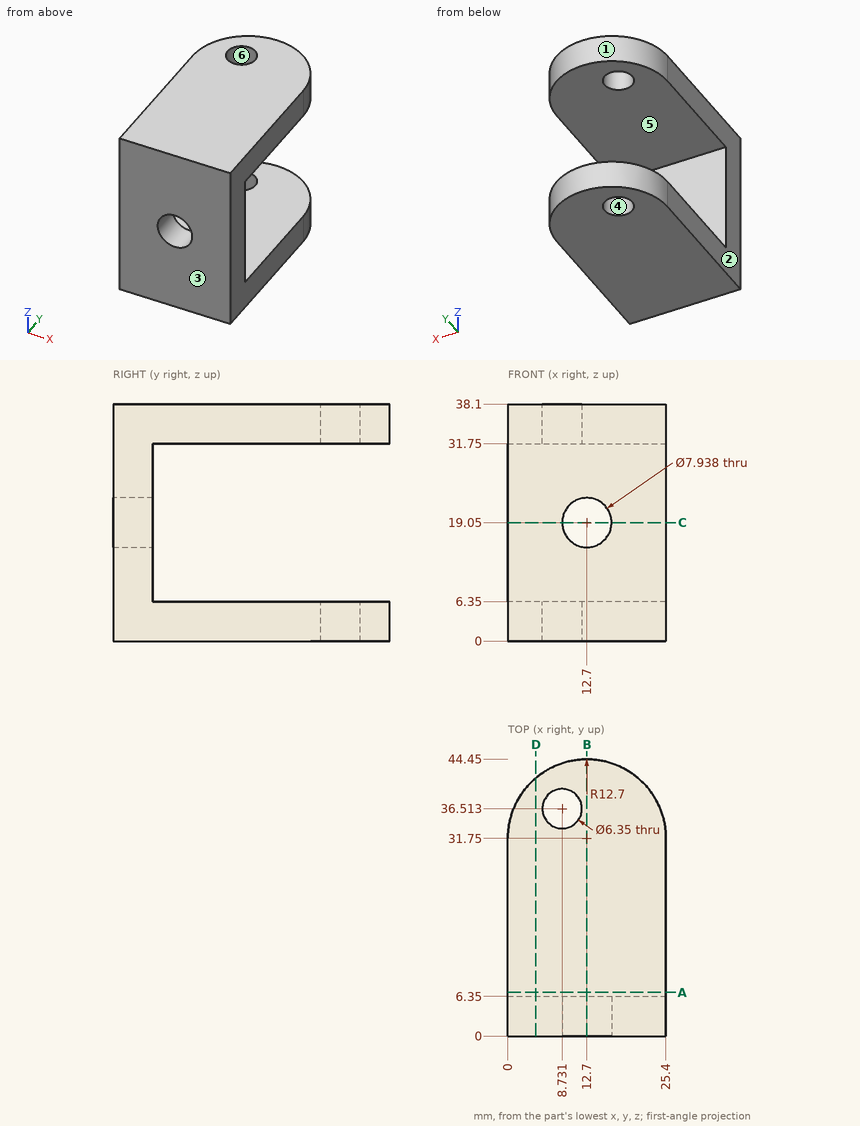
Geometry: see drawing. Coordinates: mm, zero at the bounding-box minimum. A direction names the side the tool comes from. Round coordinates to 2 decimals unless told otherwise and drop trailing zeros. Write each loop counter-clockwise with the first axis right and the second up, starting at its lowest first coordinate (ties: lowest second). Pieces come first, ordered by that corner, then holes.
1) Reachability of the marked faces 5 and 6 from +Z, -Z, +X, -X, +Y, -Y: full face, straight path, thin tool, end or side. Return the list, or none.
2) Draft query along X for the marked faces 1, 2, 3 and 4. Return one class per face: pulls with the +X half, pulls with the -X half, needs draft (parallel to the pull), parting line crosses it, or undercut.
3) Cut plane B-B (x = 12.7). Return the cut outline in (y, z).
4) Ray query, L1, parallel to Z at x = 12.25, y = 11; L2, parallel to X at y = 4.5, z = 19.05; L3, parallel to Y at x = 23, z = 24. Return the intervals inside material, ascending.
5) Cut plane C-C (z = 19.05). Return the cut outline in (x, y).
6) Contact query for a flat-ended pin moving along its axis: P1, Ø5, axis at x = 17, z = 29.5, coming from the +Y side. Output: stop coordinate, or through.
7) Cut plane D-D (x = 4.5). Return the cut outline in (y, z).
8) Cut plane A-A (y = 7). Return the cut outline in (x, z).
Geometry says:
1. face 5: +X, -X, +Y
1. face 6: +Z, -Z
2. face 1: parting line crosses it
2. face 2: pulls with the -X half
2. face 3: needs draft
2. face 4: undercut
3. outline: (0, 0) - (44.45, 0) - (44.45, 6.35) - (6.35, 6.35) - (6.35, 15.08) - (0, 15.08) - close; (0, 23.02) - (6.35, 23.02) - (6.35, 31.75) - (44.45, 31.75) - (44.45, 38.1) - (0, 38.1) - close
4. L1: z = 0 to 6.35, 31.75 to 38.1
4. L2: x = 0 to 8.73, 16.67 to 25.4
4. L3: y = 0 to 6.35
5. outline: (0, 0) - (8.73, 0) - (8.73, 6.35) - (0, 6.35) - close; (16.67, 0) - (25.4, 0) - (25.4, 6.35) - (16.67, 6.35) - close
6. P1: stops at y = 44.04
7. outline: (0, 0) - (41.45, 0) - (41.45, 6.35) - (6.35, 6.35) - (6.35, 31.75) - (41.45, 31.75) - (41.45, 38.1) - (0, 38.1) - close
8. outline: (0, 0) - (25.4, 0) - (25.4, 6.35) - (0, 6.35) - close; (0, 31.75) - (25.4, 31.75) - (25.4, 38.1) - (0, 38.1) - close
